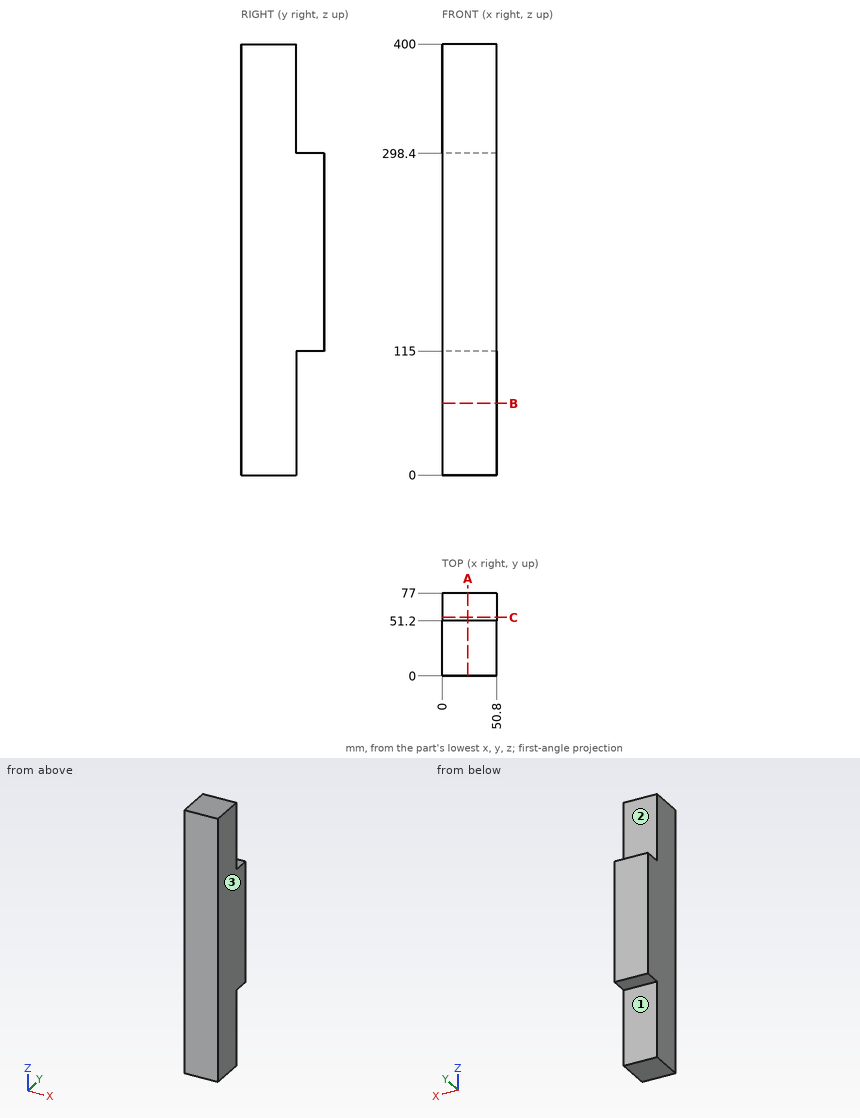
Geometry: see drawing. Coordinates: mm, zero at the bounding-box minimum. A direction names the side the tool comes from. Give positions to 0.01 mm unless a question says otherwise; leave off trailing zeros. Loops run counter-clockwise (first coordinate to the right, second up) from the corner with the lowest first, then second, coordinate; pieces in that order, holes last. Notation, with made-up numbers: (67.25, 88.25) -> (125.25, 88.25) arc R22 ccw to (125.25, 127.25) -> close; hole circle Ø5 at (75.25, -37). An arc over 180 degrees is marked (long way). Use one line per item in the form item = value.
Item 1: Pin query (flat end, axial travel): P1, Ø13, axis at x = 24, y = 60, coming from the +Z side; P2, Ø4, axis at x = 15.5, z = 52.5, coming from the +Y side. Return the tip coordinate at first contact, or that it passes through.
A:
P1 = 298.4
P2 = 51.2
Item 2: Section query C-C on y = 54.5. Output: boundary loops of the cut face in (x, z).
A:
outline = (0, 115) -> (50.8, 115) -> (50.8, 298.4) -> (0, 298.4) -> close
Item 3: Section query A-A on x = 24. Output: boundary loops of the cut face in (y, z), and give its area (3 significant figures).
A:
outline = (0, 0) -> (51.2, 0) -> (51.2, 115) -> (77, 115) -> (77, 298.4) -> (51.2, 298.4) -> (51.2, 400) -> (0, 400) -> close
area = 25,200 mm^2
Item 4: Section query B-B on z = 66.5. Output: boundary loops of the cut face in (x, y).
A:
outline = (0, 0) -> (50.8, 0) -> (50.8, 51.2) -> (0, 51.2) -> close
Item 5: Access query for the marked faces 1, 2 and 3. Directions: +Z, -Z, +X, -X, +Y, -Y. A direction counts if a zero-diameter tool reaches every point of the face in a straight line with its end or side. Return the directions, or none.
A:
face_1 = -Z, +X, -X, +Y
face_2 = +Z, +X, -X, +Y
face_3 = +Z, -Z, +X, +Y, -Y
Item 6: Line query: probe 1 along Y at (x, z) = (4, 59.5); probe 2 along Z at (x, y) = (27, 59). Output: solid intervals per line, ascending.
A:
probe_1 = 0 to 51.2
probe_2 = 115 to 298.4
